```python
from build123d import *

# Parameters (mm, degrees)
F0_W      = 41.91
F0_H      = 35.306
F1_DEPTH  = 19.05
F2_R      = 10.31875
F3_DEPTH  = 19.05
F5_DEPTH  = 14.6530745281
F6_DEPTH  = 5.842
F7_W      = 19.05
F7_H      = 4.8259994193
F8_DEPTH  = 25.4
F9_D      = 3.3
F9_DEPTH  = 12.7
F9_TIP    = 0.9914200214
F11_D     = 3.3
F12_W     = 2.444460988
F12_H     = 6.6262371838
F13_DEPTH = 59.9186
F14_DEPTH = 3.302


with BuildPart() as f1:
    # F0 (on Front) → F1 (new body)
    with BuildSketch(Plane.XZ):
        Rectangle(F0_W, F0_H)
    extrude(amount=F1_DEPTH)

    # F2 (on face) → F3 (cut, through all)
    with BuildSketch(Plane.XZ.offset(19.05)):
        with Locations((0, -6.465669493)):
            Circle(F2_R)
    extrude(amount=-F3_DEPTH, mode=Mode.SUBTRACT)

    # F4 (on face) → F5 (cut, through all)
    with BuildSketch(Plane.XY.offset(17.653)):
        Polygon((2.0530575572, -9.6835951077), (0, -9.6835951077), (-2.0530575572, -9.6835951077), (-4.1061151145, -13.2395951077), (-2.0530575572, -16.7955951077), (2.0530575572, -16.7955951077), (4.1061151145, -13.2395951077), align=None)
        Polygon((-2.0530575572, -8.3185), (0, -8.3185), (2.0530575572, -8.3185), (4.1061151145, -4.7625), (2.0530575572, -1.2065), (-2.0530575572, -1.2065), (-4.1061151145, -4.7625), align=None)
    extrude(amount=-F5_DEPTH, mode=Mode.SUBTRACT)

    # F6 (add): a face of the model
    f6_faces = [f1.faces().sort_by_distance(p)[0] for p in [
        (0, -9.5895806435, 17.653),
    ]]
    extrude(f6_faces, amount=-F6_DEPTH)

    # F7 (on face) → F8 (join)
    with BuildSketch(Plane.YZ.offset(20.955)):
        with Locations((-9.525, 15.2400002904)):
            Rectangle(F7_W, F7_H)
    extrude(amount=-F8_DEPTH)

    # F9
    with Locations(Plane.XY.offset(17.653)):
        with Locations((0, -4.7625), (0, -13.2395951077)):
            Hole(F9_D / 2, depth=F9_DEPTH)
            with Locations((0, 0, -(F9_DEPTH + F9_TIP / 2))):  # 118° drill point
                Cone(0, F9_D / 2, F9_TIP, mode=Mode.SUBTRACT)

    # F11 (through all)
    with Locations(Plane(origin=(0, 0, 0), x_dir=(-1, 0, 0), z_dir=(0, 1, 0))):
        with Locations((-13.49375, -6.465669493), (13.49375, -6.465669493)):
            Hole(F11_D / 2)

    # F12 (on face) → F13 (cut)
    with BuildSketch(Plane(origin=(-20.955, 0, 0), x_dir=(0, -1, 0), z_dir=(-1, 0, 0))):
        with Locations((10.960043408, -5.9355609119)):
            Rectangle(F12_W, F12_H)
    extrude(amount=-F13_DEPTH, mode=Mode.SUBTRACT)

    # F14 (add): a face of the model
    f14_faces = [f1.faces().sort_by_distance(p)[0] for p in [
        (0, -9.525, -17.653),
    ]]
    extrude(f14_faces, amount=F14_DEPTH)


solid = f1.part
```
Can you work these out from the model? Positions are in its coordinate system, mm. A direction names the side the tool comes from. Give positions to 0.01 mm unless a question says otherwise; leave off trailing zeros. Write each loop counter-clockwise with the first axis right and the second up, starting at its lowest first coordinate (ties: lowest second). Pieces come first, ordered by that corner, then holes. Notation, with made-up numbers: (75, 79.25) -> (108, 79.25) arc R13 cw to (108, 83.25) -> close; hole circle Ø2 at (12.5, 55). An arc over 180 degrees is marked (long way). One line per item, written item: value.
Q1. Imagine slicing it at B-B on z = -3.5. Please give me the cut outline in (x, y) (3 decimals).
Results found:
outline: (-20.955, -19.05) -> (-9.883, -19.05) -> (-9.883, -12.182) -> (-20.955, -12.182) -> close; (-20.955, -9.738) -> (-9.883, -9.738) -> (-9.883, 0) -> (-20.955, 0) -> close; (9.883, -19.05) -> (20.955, -19.05) -> (20.955, -12.182) -> (9.883, -12.182) -> close; (9.883, -9.738) -> (20.955, -9.738) -> (20.955, 0) -> (9.883, 0) -> close
Q2. Imagine slicing it at A-A on x = 0. Give the number of separate pieces and of enclosed holes in the cut face, and give its area (3 significant figures).
Results found:
separate pieces: 4
enclosed holes: 0
area: 183 mm^2
Q3. Please list where these lines run through material, in increasing order: line 1 (Y direction, x = 0, z = 14); line 2 (X direction, y = -17, z = 3) (3 decimals); line 3 (X direction, y = -17.75, z = -7) (3 decimals). Write a range as [from, to].
Results found:
line 1: y = [-19.05, -14.89], [-11.59, -6.41], [-3.11, 0]
line 2: x = [-20.955, -4.108], [4.108, 20.955]
line 3: x = [-20.955, -15.055], [-11.933, -10.305], [10.305, 11.933], [15.055, 20.955]
Q4. We'd pull the mould along Y, two halves only. Please class faces 5 (the face through (-15.3, -12.182, -6)), 6 (the face through (-3.094, -14.993, 7.983)), 7 (the face through (11.845, -4.937, -6.393)), 8 (the face through (-5, -19.05, 3)): +Y half, -Y half, draft (parallel to the pull), parting line (faces both ways), or undercut.
Results found:
face 5: undercut
face 6: undercut
face 7: draft
face 8: -Y half
Q5. Which directions (+Z, -Z, +X, -X, +Y, -Y) give clear straight access to the entire face, cutting with the end or side of a thin tool? Please do faces 1 (the face through (-15, -11, -2.622)), 2 (the face through (0, -9, 17.653)), 3 (the face through (0.358, -6.373, 15.206)), 4 (the face through (-3.065, -2.96, 7.983)).
Results found:
face 1: +X, -X
face 2: +Z, +X, -X, +Y, -Y
face 3: +Z
face 4: none
